```python
from build123d import *

# Parameters (mm, degrees)
BOSS_EXTRUDE1_DEPTH = 29.057599999999997
SKETCH3_R           = 3.4290000000000025
CUT_EXTRUDE2_DEPTH  = 40.78888094416812
SKETCH3_3_W         = 15.239999999999998
SKETCH3_3_H         = 3.8099999999999987
SKETCH3_3_W_2       = 15.239999999999997
SKETCH3_3_H_2       = 3.8100000000000014
BOSS_EXTRUDE2_DEPTH = 2.54
SKETCH2_R           = 2.6161999999999974
CUT_EXTRUDE1_DEPTH  = 46.51431433261163
FILLET7_R           = 5.08
FILLET8_R           = 7.619999999999999
SKETCH4_R           = 5.08
CUT_EXTRUDE3_DEPTH  = 10.16
FILLET9_R           = 5.08


with BuildPart() as part:
    # Sketch1 → Boss-Extrude1 (new body)
    with BuildSketch(Plane.XY):
        Polygon((0, 0), (0, 4.826), (17.91179216878401, 4.825999999999999), (27.250871205961722, -15.201719626413484), (25.29415269374959, -16.114152453511647), (17.779999999999998, 7.8e-16), align=None)
    extrude(amount=BOSS_EXTRUDE1_DEPTH)

    # Sketch3 → Cut-Extrude2 (cut, through all)
    with BuildSketch(Plane(origin=(14.604381850113365, 6.810135099327686, 0), x_dir=(0.4226182617406973, -0.9063077870366509, 0), z_dir=(-0.906307787036651, -0.42261826174069733, 0))):
        with Locations((17.674152693749598, 14.528799999999999)):
            Circle(SKETCH3_R)
    extrude(amount=-CUT_EXTRUDE2_DEPTH, mode=Mode.SUBTRACT)

    # Sketch3_3 → Boss-Extrude2 (add)
    with BuildSketch(Plane(origin=(14.604381850113365, 6.810135099327686, 0), x_dir=(0.4226182617406973, -0.9063077870366509, 0), z_dir=(-0.906307787036651, -0.42261826174069733, 0))):
        with Locations((17.67415269374959, 19.8628)):
            Rectangle(SKETCH3_3_W, SKETCH3_3_H)
        with Locations((17.674152693749594, 9.194799999999997)):
            Rectangle(SKETCH3_3_W_2, SKETCH3_3_H_2)
    extrude(amount=BOSS_EXTRUDE2_DEPTH)

    # Sketch2 → Cut-Extrude1 (cut, through all)
    with BuildSketch(Plane(origin=(2.3e-16, 4.826, 0), x_dir=(1, 0, 0), z_dir=(0, 1, 0))):
        with Locations(Location((8.955896084392007, -5.079999999999997, 0), (0, 0, 270))):
            Circle(SKETCH2_R)
        with Locations(Location((8.955896084392007, -23.9776, 0), (0, 0, 270))):
            Circle(SKETCH2_R)
    extrude(amount=-CUT_EXTRUDE1_DEPTH, mode=Mode.SUBTRACT)

    # Fillet7
    fillet7_edges = [part.edges().sort_by_distance(p)[0] for p in [
        (0, 2.413, 29.057599999999997),
        (0, 2.413, 0),
    ]]
    fillet(fillet7_edges, radius=FILLET7_R)

    # Fillet8
    fillet8_edges = [part.edges().sort_by_distance(p)[0] for p in [
        (26.272511949855655, -15.657936039962564, 0),
        (26.272511949855655, -15.657936039962564, 29.057599999999997),
    ]]
    fillet(fillet8_edges, radius=FILLET8_R)

    # Sketch4 → Cut-Extrude3 (cut)
    with BuildSketch(Plane(origin=(2.3e-16, 4.826, 0), x_dir=(1, 0, 0), z_dir=(0, 1, 0))):
        with Locations((0, -14.528799999999999)):
            Circle(SKETCH4_R)
    extrude(amount=-CUT_EXTRUDE3_DEPTH, mode=Mode.SUBTRACT)

    # Fillet9
    fillet9_edges = [part.edges().sort_by_distance(p)[0] for p in [
        (0, 2.413, 19.6088),
        (0, 2.413, 9.448799999999999),
    ]]
    fillet(fillet9_edges, radius=FILLET9_R)


solid = part.part
```
CAD build for the part. Positions are in the model's coordinates, mm. A direction names the side the tool comes from. Coordinates: 2 decimals unless noted, no trailing zeros. Write each loop counter-clockwise with the first axis right and the second up, starting at its lowest first coordinate (ties: lowest second). Pieces come first, ordered by that corner, then holes.
(1) Cut at D-D, the plane z = 27. List the corners of the cut face in (x, y).
(2) Flat gauge pins, fed straight in: pin 1 (3 mm diameter, centred on x = 8.96, z = 5.08, fed in from -Y); pin 2 (9 mm diameter, centred on x = 8.5, z = 17, fed in from -Y); pin 3 (7 mm diameter, centred on x = 20, y = -7.5, fed in from +Z); pin 4 (2 mm diameter, centred on x = 23.5, z = 19.5, fed in from +Y). Where does each tip first touch, or does it go through?
(3) Cut at C-C, the plane z = 11.75. List the corners of the cut face in (x, y).
(4) Two-plate mould, pull along Y, no slides. Class faces 1 (the face through (14.6, 0.4, 0)), 2 (the face through (17.72, -2.83, 19.84)), 3 (the face through (24.4, -14.2, 14.5)): +Y half, -Y half, draft (parallel to the pull), parting line (faces both ways), or undercut.
(5) 3-axis set-ups, long thin cutter, end or side, ignore diameter. For faces 4 (the face through (11.55, 2.45, 4.74)), 5 (the face through (21, -10, 21.768)), 6 (the face through (21, -10, 17.958)): which of +Z, -Z, +X, -X, +Y, -Y reach the whole face in a straight line?
(6) Cut at B-B, the plane x = 3.5. List the corners of the cut face in (y, z), and give its area (3 significant figures).
(7) Cut at A-A, the plane z = 6.5. List the corners of the cut face in (x, y), and give its area (3 significant figures).
(8) Drill centre lines: probe 1 along Z at (x, y) = (21, -12.25); probe 2 along Y at (x, z) = (8.5, 26.75); probe 3 along X at (y, z) = (1, 5.08). Where is each one in solid material? Low to high.
Geometry says:
1. outline: (1, 0) - (17.78, 0) - (24.27, -13.93) - (26.23, -13.02) - (17.91, 4.83) - (1, 4.83) - close
2. pin 1: passes through
2. pin 2: stops at y = 0
2. pin 3: stops at z = 29.06
2. pin 4: stops at y = -5.01
3. outline: (4.25, 0) - (17.78, 0) - (21.22, -7.39) - (23.18, -6.47) - (17.91, 4.83) - (4.25, 4.83) - close; (22.92, -11.03) - (25.29, -16.11) - (27.25, -15.2) - (24.88, -10.12) - close
4. face 1: draft
4. face 2: undercut
4. face 3: -Y half
5. face 4: +Y, -Y
5. face 5: +Z, -X, -Y
5. face 6: -X, -Y
6. outline: (0, 0.25) - (4.83, 0.25) - (4.83, 10.85) - (0, 10.85) - close; (0, 18.21) - (4.83, 18.21) - (4.83, 28.81) - (0, 28.81) - close
6. area: 102 mm2
7. outline: (0.06, 0) - (6.76, 0) - (6.76, 4.83) - (0.06, 4.83) - close; (11.15, 0) - (17.78, 0) - (25.26, -16.04) - (27.22, -15.13) - (17.91, 4.83) - (11.15, 4.83) - close
7. area: 108 mm2
8. probe 1: z = 7.29 to 11.1, 17.96 to 21.77
8. probe 2: y = 0 to 4.83
8. probe 3: x = 0 to 6.34, 11.57 to 19.7
